Read the model definition and answer for the solid it produces. Units are mm, in the model's axes. Give positions to 0.01 mm unless a question says otherwise; leave off trailing zeros. Order: outer loops, then holes, each group sorted by start corner. A loop starts at its lowest first (then second) coordinate and runs counter-clockwise, first axis right, second up. Notation, with made-up numbers: (-5, -6.75) - (7, -6.75) arc R9 ccw to (7, 5.25) - close; hole circle Ø10 at (13.5, 83). An arc over 180 degrees is marked (long way). Write each question's results on one line, items separated by ' | '.
from build123d import *

# Parameters (mm, degrees)
SKETCH1_W           = 18
SKETCH1_H           = 7
BOSS_EXTRUDE1_DEPTH = 390
SKETCH3_R           = 1.5
CUT_EXTRUDE1_DEPTH  = 390
CUT_EXTRUDE2_DEPTH  = 390


with BuildPart() as part:
    # Sketch1 → Boss-Extrude1 (new body)
    with BuildSketch(Plane.XY):
        Rectangle(SKETCH1_W, SKETCH1_H)
    extrude(amount=BOSS_EXTRUDE1_DEPTH)

    # Sketch3 → Cut-Extrude1 (cut)
    with BuildSketch(Plane(origin=(0, 3.5, 0), x_dir=(1, 0, 0), z_dir=(0, 1, 0))):
        with Locations((0, -13)):
            Circle(SKETCH3_R)
        with Locations((0, -43)):
            Circle(SKETCH3_R)
        with Locations((0, -73)):
            Circle(SKETCH3_R)
        with Locations((0, -103)):
            Circle(SKETCH3_R)
        with Locations((0, -133)):
            Circle(SKETCH3_R)
        with Locations((0, -163)):
            Circle(SKETCH3_R)
        with Locations((0, -193)):
            Circle(SKETCH3_R)
        with Locations((0, -223)):
            Circle(SKETCH3_R)
        with Locations((0, -253)):
            Circle(SKETCH3_R)
        with Locations((0, -283)):
            Circle(SKETCH3_R)
        with Locations((0, -313)):
            Circle(SKETCH3_R)
        with Locations((0, -343)):
            Circle(SKETCH3_R)
        with Locations((0, -373)):
            Circle(SKETCH3_R)
    extrude(amount=-CUT_EXTRUDE1_DEPTH, mode=Mode.SUBTRACT)

    # Sketch5 → Cut-Extrude2 (cut)
    with BuildSketch(Plane(origin=(0, 0, 0), x_dir=(-1, 0, 0), z_dir=(0, 0, -1))):
        Polygon((-9, 1.5), (-9, -0.5), (-7.5, 0.5), align=None)
        Polygon((9, -0.5), (9, 1.5), (7.5, 0.5), align=None)
    extrude(amount=-CUT_EXTRUDE2_DEPTH, mode=Mode.SUBTRACT)


solid = part.part
(1) Consider probe 1 along X at (y, z) = (2, 283); probe 2 along X at (y, z) = (0.5, 111.5); probe 3 along X at (y, z) = (0.25, 163) (3 decimals). Determine where each line is inside the solid, lowest interval first. Write a range as [from, to].
Conclusion:
probe 1: [-9, -1.5], [1.5, 9] | probe 2: [-7.5, 7.5] | probe 3: [-7.875, -1.5], [1.5, 7.875]
(2) The mould has two halves that part along Z. Classify faces 1 (the face through (0, 0, 0)), 2 (the face through (0, 0, 390)), 3 (the face through (-2, -3.5, 192)): pulls with the +Z half, pulls with the -Z half, needs draft (parallel to the pull), parting line crosses it, or undercut.
Conclusion:
face 1: pulls with the -Z half | face 2: pulls with the +Z half | face 3: needs draft
(3) Section A-A (z = 187.5) is taken. Give the vertices of the cut face in (x, y).
Conclusion:
outline: (-9, -3.5) - (9, -3.5) - (9, -0.5) - (7.5, 0.5) - (9, 1.5) - (9, 3.5) - (-9, 3.5) - (-9, 1.5) - (-7.5, 0.5) - (-9, -0.5) - close
